```python
from build123d import *

# Parameters (mm, degrees)
CROQUIS1_R              = 5.9
SALIENTE_EXTRUIR1_DEPTH = 40
CROQUIS2_R              = 5.4
SALIENTE_EXTRUIR2_DEPTH = 14.25
CROQUIS3_R              = 5.125
SALIENTE_EXTRUIR3_DEPTH = 1.2
CROQUIS4_R              = 2.8
SALIENTE_EXTRUIR4_DEPTH = 5
CROQUIS6_R              = 5.25
SALIENTE_EXTRUIR6_DEPTH = 5


with BuildPart() as part:
    # Croquis1 → Saliente-Extruir1 (new body)
    with BuildSketch(Plane(origin=(0, 0, 0), x_dir=(1, 0, 0), z_dir=(0, 1, 0))):
        with Locations(Location((0, 0, 0), (0, 0, 270))):
            Circle(CROQUIS1_R)
    extrude(amount=SALIENTE_EXTRUIR1_DEPTH)

    # Croquis2 → Saliente-Extruir2 (add)
    with BuildSketch(Plane(origin=(0, 40, 0), x_dir=(1, 0, 0), z_dir=(0, 1, 0))):
        with Locations(Location((0, 0, 0), (0, 0, 90))):
            Circle(CROQUIS2_R)
    extrude(amount=SALIENTE_EXTRUIR2_DEPTH)

    # Croquis3 → Saliente-Extruir3 (add)
    with BuildSketch(Plane(origin=(0, 54.25, 0), x_dir=(1, 0, 0), z_dir=(0, 1, 0))):
        with Locations(Location((0, 0, 0), (0, 0, 270))):
            Circle(CROQUIS3_R)
    extrude(amount=SALIENTE_EXTRUIR3_DEPTH)

    # Croquis4 → Saliente-Extruir4 (add)
    with BuildSketch(Plane(origin=(0, 55.45, 0), x_dir=(1, 0, 0), z_dir=(0, 1, 0))):
        with Locations(Location((0, -2.325, 0), (0, 0, 270))):
            Circle(CROQUIS4_R)
    extrude(amount=SALIENTE_EXTRUIR4_DEPTH)

    # Croquis6 → Saliente-Extruir6 (add)
    with BuildSketch(Plane.XZ):
        with Locations(Location((0, 0, 0), (0, 0, 90))):
            Circle(CROQUIS6_R)
    extrude(amount=SALIENTE_EXTRUIR6_DEPTH)

    # Croquis7 → Revolución1 (revolve)
    with BuildSketch(Plane(origin=(0, 55.45, 0), x_dir=(1, 0, 0), z_dir=(0, 1, 0))):
        with BuildLine():
            Line((0, 2.5), (0, 4.5))
            ThreePointArc((0, 4.5), (-1, 3.5), (0, 2.5))
        make_face()
    revolve(axis=Axis((0, 55.45, -2.5), (0, 0, -1)))


solid = part.part
```
For this review, take the finished solid that the model builds, in its own axes (mm). A direction names the side the tool comes from. Round coordinates to 2 decimals unless told otherwise and drop trailing zeros. Loops run counter-clockwise (first coordinate to the right, second up) from the corner with the lowest first, then second, coordinate; pieces in that order, holes last.
(1) We need section D-D (x = 3.75). Give the boundary of the cut face in (y, z).
Returned:
outline: (-5, -3.67) - (0, -3.67) - (0, -4.55) - (40, -4.55) - (40, -3.89) - (54.25, -3.89) - (54.25, -3.49) - (55.45, -3.49) - (55.45, 3.49) - (54.25, 3.49) - (54.25, 3.89) - (40, 3.89) - (40, 4.55) - (0, 4.55) - (0, 3.67) - (-5, 3.67) - close
(2) Wall thickness on line 1 along Y through (x, z) = (2, 4.5); line 2 along X through (y, z) = (25, 3); line 3 along Z through (x, y) = (3.75, 5): over which ranges is each line inside the solid? List them lowest first.
Returned:
line 1: y = -5 to 55.45
line 2: x = -5.08 to 5.08
line 3: z = -4.55 to 4.55
(3) Mouldability with a two-part tool opening along Y and no side actions: class faces 4 (the flat face through (0, 55.45, -1)), 5 (the cylindrical face through (-5.003, 54.842, -1.111)), 6 (the flat face through (-4, 0, -4)) as released by +Y, released by -Y, zero draft, split by the parting line, or undercut.
Returned:
face 4: released by +Y
face 5: zero draft
face 6: released by -Y
(4) Clearance check with flat-ended pins moving along their axes: P1, Ø1.5, axis at x = -3, y = 39, coming from the -Z side; P2, Ø1, axis at x = 2, y = 9, coming from the -Z side; P3, Ø6, axis at y = 45.5, z = -1.5, coming from the -X side. State where each tip first meets the part, or that it passes through.
Returned:
P1: stops at z = -5.45
P2: stops at z = -5.71
P3: stops at x = -5.4
(5) We need section B-B (z = 3.5). Give the boundary of the cut face in (x, y).
Returned:
outline: (-4.75, 0) - (-3.91, 0) - (-3.91, -5) - (3.91, -5) - (3.91, 0) - (4.75, 0) - (4.75, 40) - (4.11, 40) - (4.11, 54.25) - (3.74, 54.25) - (3.74, 55.45) - (2.54, 55.45) - (2.54, 60.45) - (-2.54, 60.45) - (-2.54, 55.45) - (-3.74, 55.45) - (-3.74, 54.25) - (-4.11, 54.25) - (-4.11, 40) - (-4.75, 40) - close
(6) We need section A-A (x = -4). Give the boundary of the cut face in (y, z).
Returned:
outline: (-5, -3.4) - (0, -3.4) - (0, -4.34) - (40, -4.34) - (40, -3.63) - (54.25, -3.63) - (54.25, -3.2) - (55.45, -3.2) - (55.45, 3.2) - (54.25, 3.2) - (54.25, 3.63) - (40, 3.63) - (40, 4.34) - (0, 4.34) - (0, 3.4) - (-5, 3.4) - close
(7) Tool access review of faces 1 (the flat face through (0, 60.45, 2)), 2 (the cylindrical face through (-1.6, -2.5, 5)), 3 (the cylindrical face through (0.123, 57.915, -0.472)): name each direction out of +Z, -Z, +X, -X, +Y, -Y from which nothing blocks a thin tool from reaching the whole face with its end or side.
Returned:
face 1: +Z, -Z, +X, -X, +Y
face 2: -Y
face 3: +Y
(8) We need section C-C (y = 50.5). Give the boundary of the cut face in (x, z).
Returned:
outline: circle Ø10.8 at (0, 0)
